Verification items for the finished model (mm, model axes). A direction names the side the tool comes from. Coordinates: 2 decimals unless noted, no trailing zeros. Order: outer loops, then holes, each group sorted by start corner. A loop starts at its lowest first (then second) coordinate and runs counter-clockwise, first axis right, second up. Notation, with made-up numbers: M 84,-9 L 94,-9 A14 cw 94,2 Z; hole C 40.5,-6.75 d2. An arc over 180 degrees is marked long. Answer as a JSON object with one key per item and string values. Group by question number.
(1) Cross-section at D-D (x = -4.5). Enter the section's corners in (y, z).
(2) Cross-section at A-A (y = 0). Enter the section's corners in (x, z), plus the area to 3 significant figures.
(3) Material ranges on line 1 (Z direction, x = -4.9, y = 0); line 2 (Z direction, x = -6, y = 1); line 3 (X direction, y = 0, z = 11.25), recorded low to high.
(4) Mould release check, pull along Z, two halves, no side actions. Record for faces 1 (the face through (3, 3, 26.988)), 2 (the face through (-5.012, 0.5, 23.576)), 3 (the face through (5.95, -3.45, 0.38)), 4 (the face through (-5.012, 0.5, 15.575)): released by +Z, released by -Z, zero draft, split by the parting line, or undercut.
(5) Gauge pin test, flat ends, axial feed: pin 1 Ø4 at (x, y) = (-1, -1) entering from +Z; pin 2 Ø2 at (x, z) = (-0.5, 9.5) entering from +Y. Record the tip position at first contact, or that the pin passes through.
(6) Cross-section at C-C (x = 0). Enter the section's corners in (y, z).
(7) Access from +Z, -Z, +X, -X, +Y, -Y to the whole of each face (thin tool, end or side, straight path). Record for faces 5 (the face through (3.695, -1.532, 17.128)), 6 (the face through (-3.14, 5.52, 0.38)).
(8) Cross-section at B-B (z = 7.5). Enter the section's corners in (x, y).
from build123d import *

# Parameters (mm, degrees)
SKETCH1_R               = 6.35
BASIC_ROD_DEPTH         = 26.9875
BASIC_ROD_DEPTH_BACK    = 26.9875
THEX_DEPTH              = 26.9875
SKETCH2_R               = 2.11582
INTERNAL_CUT_DEPTH      = 27.9875
INTERNAL_CUT_DEPTH_BACK = 27.9875
SKETCH9_R               = 4
CUT_EXTRUDE1_DEPTH      = 19.99996
CUT_EXTRUDE2_REACH      = 14.7
SKETCH10_R              = 1.66624


with BuildPart() as part:
    # Sketch1 → Basic Rod (new body, two sides)
    with BuildSketch(Plane.XY) as basic_rod_sk:
        Circle(SKETCH1_R)
    extrude(amount=BASIC_ROD_DEPTH)
    extrude(basic_rod_sk.sketch, amount=-BASIC_ROD_DEPTH_BACK)

    # Sketch8 → THex (add, symmetric)
    with BuildSketch(Plane.XY):
        with BuildLine():
            Line((-0.888411378, 6.819423871), (-5.461588622, 4.179098758))
            ThreePointArc((-5.461588622, 4.179098758), (-5.955700003, 3.438525), (-6.35, 2.640325113))
            Line((-6.35, 2.640325113), (-6.35, -2.640325113))
            ThreePointArc((-6.35, -2.640325113), (-5.955700003, -3.438525), (-5.461588622, -4.179098758))
            Line((-5.461588622, -4.179098758), (-0.888411378, -6.819423871))
            ThreePointArc((-0.888411378, -6.819423871), (0, -6.87705), (0.888411378, -6.819423871))
            Line((0.888411378, -6.819423871), (5.461588622, -4.179098758))
            ThreePointArc((5.461588622, -4.179098758), (5.955700003, -3.438525), (6.35, -2.640325113))
            Line((6.35, -2.640325113), (6.35, 2.640325113))
            ThreePointArc((6.35, 2.640325113), (5.955700003, 3.438525), (5.461588622, 4.179098758))
            Line((5.461588622, 4.179098758), (0.888411378, 6.819423871))
            ThreePointArc((0.888411378, 6.819423871), (0, 6.87705), (-0.888411378, 6.819423871))
        make_face()
    extrude(amount=THEX_DEPTH, both=True)

    # Sketch2 → Internal Cut (cut, two sides)
    with BuildSketch(Plane.XY) as internal_cut_sk:
        Circle(SKETCH2_R)
    extrude(amount=INTERNAL_CUT_DEPTH, mode=Mode.SUBTRACT)
    extrude(internal_cut_sk.sketch, amount=-INTERNAL_CUT_DEPTH_BACK, mode=Mode.SUBTRACT)

    # Sketch9 → Cut-Extrude1 (cut)
    with BuildSketch(Plane.XY.offset(26.9875)):
        Circle(SKETCH9_R)
    extrude(amount=-CUT_EXTRUDE1_DEPTH, mode=Mode.SUBTRACT)

    # Sketch10 → Cut-Extrude2 (cut, up to next)
    with BuildSketch(Plane.ZY.offset(6.35), mode=Mode.PRIVATE) as cut_extrude2_sk1:
        with Locations((13.98524, 0)):
            Circle(SKETCH10_R)
    cut_extrude2_tool1 = extrude(cut_extrude2_sk1.sketch, amount=-CUT_EXTRUDE2_REACH, mode=Mode.PRIVATE) & part.part
    add(cut_extrude2_tool1.solids().sort_by_distance((-6.35, 0, 13.98524))[0], mode=Mode.SUBTRACT)
    # Sketch10 → Cut-Extrude2 (cut, up to next)
    with BuildSketch(Plane.ZY.offset(6.35), mode=Mode.PRIVATE) as cut_extrude2_sk2:
        with Locations((21.98624, 0)):
            Circle(SKETCH10_R)
    cut_extrude2_tool2 = extrude(cut_extrude2_sk2.sketch, amount=-CUT_EXTRUDE2_REACH, mode=Mode.PRIVATE) & part.part
    add(cut_extrude2_tool2.solids().sort_by_distance((-6.35, 0, 21.98624))[0], mode=Mode.SUBTRACT)


solid = part.part
Taken from the geometry:
{
 "1": {"outline": "M -4.73,-26.99 L 4.73,-26.99 L 4.73,26.99 L -4.73,26.99 Z; hole C 0,13.99 d3.33; hole C 0,21.99 d3.33"},
 "2": {"outline": "M -6.35,-26.99 L -2.12,-26.99 L -2.12,6.99 L -4,6.99 L -4,12.32 L -6.35,12.32 Z; M -6.35,15.65 L -4,15.65 L -4,20.32 L -6.35,20.32 Z; M -6.35,23.65 L -4,23.65 L -4,26.99 L -6.35,26.99 Z; M 2.12,-26.99 L 6.35,-26.99 L 6.35,26.99 L 4,26.99 L 4,6.99 L 2.12,6.99 Z", "area": "366 mm²"},
 "3": {"line 1": "z = -26.99 to 12.32, 15.65 to 20.32, 23.65 to 26.99", "line 2": "z = -26.99 to 12.65, 15.32 to 20.65, 23.32 to 26.99", "line 3": "x = -6.35 to -4, 4 to 6.35"},
 "4": {"face 1": "released by +Z", "face 2": "undercut", "face 3": "zero draft", "face 4": "undercut"},
 "5": {"pin 1": "stops at z = 6.99", "pin 2": "stops at y = 6.88"},
 "6": {"outline": "M -6.88,-26.99 L -2.12,-26.99 L -2.12,6.99 L -4,6.99 L -4,26.99 L -6.88,26.99 Z; M 2.12,-26.99 L 6.88,-26.99 L 6.88,26.99 L 4,26.99 L 4,6.99 L 2.12,6.99 Z"},
 "7": {"face 5": "+Z", "face 6": "+Z, -Z, -X, +Y"},
 "8": {"outline": "M -6.35,-2.64 A6.88 ccw -5.46,-4.18 L -0.89,-6.82 A6.88 ccw 0.89,-6.82 L 5.46,-4.18 A6.88 ccw 6.35,-2.64 L 6.35,2.64 A6.88 ccw 5.46,4.18 L 0.89,6.82 A6.88 ccw -0.89,6.82 L -5.46,4.18 A6.88 ccw -6.35,2.64 Z; hole C 0,0 d8"}
}
